from build123d import *

# Parameters (mm, degrees)
BOSS_EXTRUDE1_DEPTH      = 457.2
BOSS_EXTRUDE1_DEPTH_BACK = 457.2
SKETCH3_W                = 63.5
SKETCH3_H                = 31.75
SKETCH3_W_2              = 57.15
SKETCH3_H_2              = 25.4
SKETCH5_R                = 3.571875
CUT_EXTRUDE1_DEPTH       = 460.399570091
SKETCH8_R                = 3.57251
CUT_EXTRUDE2_DEPTH       = 460.399570091


with BuildPart() as part:
    # Sketch3 → Boss-Extrude1 (new, two sides: drawn at the far end of the back side and taken through both)
    with BuildSketch(Plane.XY.offset(-BOSS_EXTRUDE1_DEPTH_BACK)):
        Rectangle(SKETCH3_W, SKETCH3_H)
        Rectangle(SKETCH3_W_2, SKETCH3_H_2, mode=Mode.SUBTRACT)
    extrude(amount=BOSS_EXTRUDE1_DEPTH + BOSS_EXTRUDE1_DEPTH_BACK)

    # Sketch5 → Cut-Extrude1 (cut, through all)
    with BuildSketch(Plane.XZ.offset(15.875)):
        with Locations(Location((-22.225, 392.1125, 0), (0, 0, 270))):
            Circle(SKETCH5_R)
        with Locations(Location((22.225, 392.1125, 0), (0, 0, 270))):
            Circle(SKETCH5_R)
        with Locations(Location((22.225, -392.1125, 0), (0, 0, 90))):
            Circle(SKETCH5_R)
        with Locations(Location((-22.225, -392.1125, 0), (0, 0, 90))):
            Circle(SKETCH5_R)
        with Locations(Location((22.225, 376.2375, 0), (0, 0, 90))):
            Circle(SKETCH5_R)
        with Locations(Location((-22.225, 376.2375, 0), (0, 0, 90))):
            Circle(SKETCH5_R)
        with Locations(Location((22.225, -376.2375, 0), (0, 0, 270))):
            Circle(SKETCH5_R)
        with Locations(Location((-22.225, -376.2375, 0), (0, 0, 270))):
            Circle(SKETCH5_R)
    extrude(amount=-CUT_EXTRUDE1_DEPTH, mode=Mode.SUBTRACT)

    # Sketch8 → Cut-Extrude2 (cut, through all)
    with BuildSketch(Plane(origin=(0, 15.875, 0), x_dir=(1, 0, 0), z_dir=(0, 1, 0))):
        with Locations(Location((21.772898576, 228.6, 0), (0, 0, 180))):
            Circle(SKETCH8_R)
        with Locations(Location((-22.677101424, 228.6, 0), (0, 0, 180))):
            Circle(SKETCH8_R)
        with Locations(Location((21.772898576, -228.6, 0), (0, 0, 270))):
            Circle(SKETCH8_R)
        with Locations(Location((-22.677101424, -228.6, 0), (0, 0, 270))):
            Circle(SKETCH8_R)
    extrude(amount=-CUT_EXTRUDE2_DEPTH, mode=Mode.SUBTRACT)


solid = part.part
Could you check a few things on this model? Use its own coordinates, in mm. A direction names the side the tool comes from. Coordinates: 2 decimals unless noted, no trailing zeros. Order: outer loops, then holes, each group sorted by start corner. A loop starts at its lowest first (then second) coordinate and runs counter-clockwise, first axis right, second up. Notation, with made-up numbers: (-39, 21) -> (-23, 21) arc R23 ccw to (-23, 55) -> close; hole circle Ø7 at (89, 60.5). An arc over 180 degrees is marked (long way). One line per item, written item: value. Start each with the question number.
1) Imagine slicing it at A-A on x = 1.5. List the corners of the cut face in (y, z) for me (3 decimals), plus the area to 3 significant figures.
2) Imagine slicing it at B-B on y = 6. List the corners of the cut face in (x, z) for me (3 decimals).
3) We'd pull the mould along Y, two halves only. Please class faces 3 (the flat face through (-28.575, 0, -6)), 4 (the flat face through (0, 15.875, -6)), 5 (the flat face through (0, -15.875, -6)): +Y half, -Y half, draft (parallel to the pull), parting line (faces both ways), or undercut.
4) Imagine slicing it at C-C on z = 128. List the corners of the cut face in (x, y) for me (3 decimals), plus the area to 3 significant figures.
5) If I drill on L1, parallel to X at y = -14, z = -228; L2, parallel to X at y = 4, z = -201.5 (3 decimals); L3, parallel to Y at x = -14, z = -129 (3 decimals), over which ranges is the centre line in solid material (lowest first)? Write a range as [from, to].
6) I'm going to push flat-ended pins straight in: pin 1 (4.5 mm diameter, centred on x = 22.22, z = -376.24, fed in from -Y); pin 2 (9.5 mm diameter, centred on x = 22.22, z = -376.24, fed in from -Y) (3 decimals). Where does each tip first touch, or does it pass through?
7) Which directions (+Z, -Z, +X, -X, +Y, -Y) give clear straight access to the entire face, cutting with the end or side of a thin tool? Please do faces 1 (the flat face through (31.75, 0, -6)), 2 (the flat face through (28.575, 0, -6)).
Answer list:
1. outline: (-15.875, -457.2) -> (-12.7, -457.2) -> (-12.7, 457.2) -> (-15.875, 457.2) -> close; (12.7, -457.2) -> (15.875, -457.2) -> (15.875, 457.2) -> (12.7, 457.2) -> close
1. area: 5,810 mm2
2. outline: (-31.75, -457.2) -> (-28.575, -457.2) -> (-28.575, 457.2) -> (-31.75, 457.2) -> close; (28.575, -457.2) -> (31.75, -457.2) -> (31.75, 457.2) -> (28.575, 457.2) -> close
3. face 3: undercut
3. face 4: +Y half
3. face 5: -Y half
4. outline: (-31.75, -15.875) -> (31.75, -15.875) -> (31.75, 15.875) -> (-31.75, 15.875) -> close; hole (-28.575, -12.7) -> (28.575, -12.7) -> (28.575, 12.7) -> (-28.575, 12.7) -> close
4. area: 565 mm2
5. L1: x = [-31.75, -26.2], [-19.16, 18.25], [25.29, 31.75]
5. L2: x = [-31.75, -28.575], [28.575, 31.75]
5. L3: y = [-15.875, -12.7], [12.7, 15.875]
6. pin 1: passes through
6. pin 2: stops at y = -15.875
7. face 1: +Z, -Z, +X, +Y, -Y
7. face 2: +Z, -Z
